```python
from build123d import *

# Parameters (mm, degrees)
SKETCH1_W                                         = 65
SKETCH1_H                                         = 37.4
BOSS_EXTRUDE1_DEPTH                               = 60
SKETCH2_R                                         = 15.875
CUT_EXTRUDE1_DEPTH                                = 91.41399228
F_1_0MM_DOWEL_HOLE1_D                             = 2.5
F_1_0MM_DOWEL_HOLE1_DEPTH                         = 5
F_1_0MM_DOWEL_HOLE1_TIP                           = 0.751075774
LPATTERN2_COUNT                                   = 2
LPATTERN2_PITCH                                   = 41.9
LPATTERN3_COUNT                                   = 2
LPATTERN3_PITCH                                   = 35.5
SKETCH20_R                                        = 15.875
SKETCH20_R_2                                      = 12.7
BOSS_EXTRUDE6_DEPTH                               = 7
CUT_EXTRUDE2_DEPTH                                = 4
SKETCH24_R                                        = 2
BOSS_EXTRUDE7_DEPTH                               = 8
CSK_FOR_M3_5_FLAT_HEAD_MACHINE_SCREW2_D           = 4
CSK_FOR_M3_5_FLAT_HEAD_MACHINE_SCREW2_CSINK_D     = 8.2
CSK_FOR_M3_5_FLAT_HEAD_MACHINE_SCREW2_CSINK_ANGLE = 90
F_4_0MM_DOWEL_HOLE2_D                             = 4
F_4_0MM_DOWEL_HOLE2_DEPTH                         = 4
F_4_0MM_DOWEL_HOLE2_TIP                           = 1.201721238


with BuildPart() as part:
    # Sketch1 → Boss-Extrude1 (new body)
    with BuildSketch(Plane.XY):
        Rectangle(SKETCH1_W, SKETCH1_H)
    extrude(amount=BOSS_EXTRUDE1_DEPTH)

    # Sketch2 → Cut-Extrude1 (cut, through all)
    with BuildSketch(Plane(origin=(32.5, 0, 0), x_dir=(0, 0, -1), z_dir=(1, 0, 0))):
        with Locations((-41.3, 0)):
            Circle(SKETCH2_R)
    extrude(amount=-CUT_EXTRUDE1_DEPTH, mode=Mode.SUBTRACT)

    # Ø1.0mm Dowel Hole1
    with Locations(Plane.XY.offset(60)):
        with Locations((-11, 8.07), (8.35, -14.2)):
            Hole(F_1_0MM_DOWEL_HOLE1_D / 2, depth=F_1_0MM_DOWEL_HOLE1_DEPTH)
            with Locations((0, 0, -(F_1_0MM_DOWEL_HOLE1_DEPTH + F_1_0MM_DOWEL_HOLE1_TIP / 2))):  # 118° drill point
                Cone(0, F_1_0MM_DOWEL_HOLE1_D / 2, F_1_0MM_DOWEL_HOLE1_TIP, mode=Mode.SUBTRACT)

    # Sketch19 → Ø1.0mm Dowel Hole2 (revolve, cut)
    with BuildSketch(Plane(origin=(26.5, -18.7, 54), x_dir=(0, 0, -1), z_dir=(1, 0, 0))):
        Polygon((0, 0), (0, 5.991420021), (1.65, 5), (1.65, 0), align=None)
    f_1_0mm_dowel_hole2 = revolve(axis=Axis((26.5, -25.05, 54), (0, 1, 0)), mode=Mode.SUBTRACT)

    # LPattern2: Ø1.0mm Dowel Hole2 ×2
    with Locations(*[(-i * LPATTERN2_PITCH, 0, 0) for i in range(1, LPATTERN2_COUNT)]):
        add(f_1_0mm_dowel_hole2, mode=Mode.SUBTRACT)

    # LPattern3: Ø1.0mm Dowel Hole2 ×2
    with Locations(*[(0, 0, -i * LPATTERN3_PITCH) for i in range(1, LPATTERN3_COUNT)]):
        add(f_1_0mm_dowel_hole2, mode=Mode.SUBTRACT)

    # Sketch20 → Boss-Extrude6 (add, symmetric)
    with BuildSketch(Plane(origin=(0, 0, 0), x_dir=(0, 0, -1), z_dir=(1, 0, 0))):
        with Locations((-41.3, 0)):
            Circle(SKETCH20_R)
        with Locations((-41.3, 0)):
            Circle(SKETCH20_R_2, mode=Mode.SUBTRACT)
    extrude(amount=BOSS_EXTRUDE6_DEPTH, both=True)

    # Sketch23 → Cut-Extrude2 (cut)
    with BuildSketch(Plane(origin=(32.5, 0, 0), x_dir=(0, 0, -1), z_dir=(1, 0, 0))):
        with BuildLine():
            ThreePointArc((-60, 7.092954251), (-55.442135624, 14.142135624), (-48.392954251, 18.7))
            Line((-48.392954251, 18.7), (-60, 18.7))
            Line((-60, 18.7), (-60, 7.092954251))
        make_face()
        with BuildLine():
            ThreePointArc((-48.392954251, -18.7), (-55.442135624, -14.142135624), (-60, -7.092954251))
            Line((-60, -7.092954251), (-60, -18.7))
            Line((-60, -18.7), (-48.392954251, -18.7))
        make_face()
        with BuildLine():
            Line((-13.497713028, 18.7), (-34.207045749, 18.7))
            ThreePointArc((-34.207045749, 18.7), (-21.3, 0), (-34.207045749, -18.7))
            Line((-34.207045749, -18.7), (-12.913047807, -18.7))
            add(Edge.make_bspline(
                [(-13.497713028, 18.7), (-4.48947297, 8.699685881), (-1.125683448, -8.066606066), (-12.913047807, -18.7)],
                knots=[0, 0, 0, 0, 1, 1, 1, 1], degree=3))
        make_face()
    extrude(amount=-CUT_EXTRUDE2_DEPTH, mode=Mode.SUBTRACT)

    # Sketch24 → Boss-Extrude7 (add)
    # profile 1 of 2: a face of its own
    with BuildSketch(Plane(origin=(0, 0, 0), x_dir=(-1, 0, 0), z_dir=(0, 0, -1))):
        with BuildLine():
            Line((-32.5, -18.7), (20.662392723, -18.7))
            ThreePointArc((20.662392723, -18.7), (-5.918803639, -32.5), (-32.5, -18.7))
        make_face()
        with Locations(Location((6.081196361, -24.2, 0), (0, 0, 180))):
            Circle(SKETCH24_R, mode=Mode.SUBTRACT)
        with Locations(Location((-17.918803639, -24.2, 0), (0, 0, 180))):
            Circle(SKETCH24_R, mode=Mode.SUBTRACT)
    # profile 2 of 2: a face of its own
    with BuildSketch(Plane(origin=(0, 0, 0), x_dir=(-1, 0, 0), z_dir=(0, 0, -1))):
        with BuildLine():
            Line((20.662392723, 18.7), (-32.5, 18.7))
            ThreePointArc((-32.5, 18.7), (-5.918803639, 32.5), (20.662392723, 18.7))
        make_face()
        with Locations((-17.918803639, 24.2)):
            Circle(SKETCH24_R, mode=Mode.SUBTRACT)
        with Locations((6.081196361, 24.2)):
            Circle(SKETCH24_R, mode=Mode.SUBTRACT)
    extrude(amount=-BOSS_EXTRUDE7_DEPTH)

    # CSK for M3.5 Flat Head Machine Screw2 (through all)
    with Locations(Plane.XY.offset(8)):
        with Locations((5.918803639, 28)):
            csk_for_m3_5_flat_head_machine_screw2 = CounterSinkHole(CSK_FOR_M3_5_FLAT_HEAD_MACHINE_SCREW2_D / 2, CSK_FOR_M3_5_FLAT_HEAD_MACHINE_SCREW2_CSINK_D / 2, counter_sink_angle=CSK_FOR_M3_5_FLAT_HEAD_MACHINE_SCREW2_CSINK_ANGLE)

    # Mirror1: CSK for M3.5 Flat Head Machine Screw2 across plane
    add(csk_for_m3_5_flat_head_machine_screw2.mirror(Plane.ZX), mode=Mode.SUBTRACT)

    # Ø4.0mm Dowel Hole2
    with Locations(Plane(origin=(0, 18.7, 0), x_dir=(1, 0, 0), z_dir=(0, 1, 0))):
        with Locations((-26.5, -54), (17.5, -54), (-27.64165215, -9)):
            Hole(F_4_0MM_DOWEL_HOLE2_D / 2, depth=F_4_0MM_DOWEL_HOLE2_DEPTH)
            with Locations((0, 0, -(F_4_0MM_DOWEL_HOLE2_DEPTH + F_4_0MM_DOWEL_HOLE2_TIP / 2))):  # 118° drill point
                Cone(0, F_4_0MM_DOWEL_HOLE2_D / 2, F_4_0MM_DOWEL_HOLE2_TIP, mode=Mode.SUBTRACT)


solid = part.part
```
The listing builds one solid part. Answer for the finished solid, in the listing's coordinates (mm). A direction names the side the tool comes from. Round coordinates to 2 decimals unless told otherwise and drop trailing zeros. Loops run counter-clockwise (first coordinate to the right, second up) from the corner with the lowest first, then second, coordinate; pieces in that order, holes last.
1) Given P1, Ø3, axis at x = 8.35, y = -14.2, coming from the -Z side; P2, Ø15, axis at x = -6, y = 26.5, coming from the +Z side; P3, Ø5, axis at x = -27.64, z = 9, coming from the +Y side; P4, Ø6.5, axis at x = 5.92, y = 28, coming from the +Z side, each flat-ended and moving along its own axis, determine where each tip first touches the part or whether it passes through.
Outcome:
P1: stops at z = 0
P2: stops at z = 8
P3: stops at y = 18.7
P4: stops at z = 7.15
2) Consider line 1 (X direction, y = -15.05, z = 54); line 2 (Y direction, x = -12, z = 41); line 3 (X direction, y = -18.5, z = 31.5). Determine where each line is inside the solid, lowest interval first.
Outcome:
line 1: x = -32.5 to -17.05, -13.75 to 24.85, 28.15 to 32.5
line 2: y = -18.7 to -15.87, 15.87 to 18.7
line 3: x = -32.5 to 28.5
3) A cutting plane is placed at A-A on x = 21. Determine the outline of the cut face in (y, z) (3 decimals), plus the area to 3 significant figures.
Outcome:
outline: (-28.789, 0) - (28.789, 0) - (28.789, 8) - (18.7, 8) - (18.7, 60) - (-18.7, 60) - (-18.7, 8) - (-28.789, 8) - close; hole circle Ø31.75 at (0, 41.3)
area: 1,610 mm2
4) For faces 5 (the face through (28.5, 16, 57)), 6 (the face through (6, 23, 8)), 7 (the face through (-10.84, 9.31, 57.46)), determine the directions among +Z, -Z, +X, -X, +Y, -Y from which every point of the face is accessible in a straight line to the end or side of a thin tool.
Outcome:
face 5: +Z, +X, +Y
face 6: +Z, +X, -X, +Y
face 7: +Z
5) A cutting plane is placed at B-B on x = -11. Determine the outline of the cut face in (y, z) (3 decimals), plus the area to 3 significant figures.
Outcome:
outline: (-27.749, 0) - (27.749, 0) - (27.749, 8) - (18.7, 8) - (18.7, 60) - (9.32, 60) - (9.32, 55) - (8.661, 54.604) arc R15.875 cw (long way) to (6.82, 55.635) - (6.82, 60) - (-18.7, 60) - (-18.7, 8) - (-27.749, 8) - close
area: 1,580 mm2
6) For a pull along Z with two mould halves and no side action, classify faces 1 (the face through (25.385, -16.235, 55.216)), 2 (the face through (6, -22, 8)), 3 (the face through (32.5, 0, 4)), 4 (the face through (30.528, 0.338, 21.303)) as released by +Z, released by -Z, zero draft, split by the parting line, or undercut.
Outcome:
face 1: undercut
face 2: released by +Z
face 3: zero draft
face 4: undercut
